Can you work these out from the model? Positions are in its coordinate system, mm. Round coordinates to 2 decimals unless told otherwise and drop trailing zeros. Write each loop counter-clockwise with the first axis right and the second up, starting at its lowest first coordinate (ties: lowest second). Pieces come first, ordered by that corner, then holes. Notation, with made-up numbers: (3, 21) - (42, 21) arc R18 ccw to (42, 49) - close; hole circle Ø5 at (69, 38). An arc over 180 degrees is marked (long way). One line per item, written item: value. Start each with the question number.
(1) I want a section at B-B on x = -35.5. List the corners of the cut face in (y, z) for me, plus the area to 3 significant figures.
(2) If I drill on L1, parallel to X at y = 2.4, z = -50; L2, parallel to Z at x = 51.5, y = 1.6; L3, parallel to Z at x = 17, y = 2.65, over which ranges is the centre line in solid material (lowest first)? Write a range as from..to.
(3) I want a section at A-A on y = 1.2. Give the number of separate pieces and of enclosed holes in the cut face, plus the area to 3 significant figures.
(4) I want a section at C-C on z = 21. List the corners of the cut face in (x, y) for me.
(5) I'm going to push flat-ended pins straight in: pin 1 Ø3 at (x, z) = (0, 0) entering from +Y; pin 2 Ø1 at (y, z) = (1, 41) entering from +X; pin 3 Ø1.5 at (y, z) = (1, -5.5) entering from -X; pin 4 Ø0.9 at (x, y) = (-87.5, 1) entering from -Z. Where does each tip first touch, or does it pass through?
from build123d import *

# Parameters (mm, degrees)
SKETCH_1_W            = 85
SKETCH_1_H            = 60
SKETCH_1_R            = 1.6
EXTRUDE_1_DEPTH       = 3
EXTRUDE_2_DEPTH       = 3
FILLET_1_R            = 20
FILLET_3_R            = 10
SKETCH_4_R            = 3.1
CUT_EXTRUDE_1_DEPTH   = 10
CUT_EXTRUDE_1_2_DEPTH = 10


with BuildPart() as part:
    # 草图1 → 凸台-拉伸1 (new body)
    with BuildSketch(Plane(origin=(0, 0, 0), x_dir=(1, 0, 0), z_dir=(0, 1, 0))):
        with Locations((32.5, 25)):
            Rectangle(SKETCH_1_W, SKETCH_1_H)
        with Locations(Location((0, 50, 0), (0, 0, 270))):
            Circle(SKETCH_1_R, mode=Mode.SUBTRACT)
        with Locations(Location((65, 50, 0), (0, 0, 90))):
            Circle(SKETCH_1_R, mode=Mode.SUBTRACT)
        with Locations(Location((65, 0, 0), (0, 0, 270))):
            Circle(SKETCH_1_R, mode=Mode.SUBTRACT)
        with Locations(Location((0, 0, 0), (0, 0, 90))):
            Circle(SKETCH_1_R, mode=Mode.SUBTRACT)
    extrude(amount=EXTRUDE_1_DEPTH)

    # 草图2 → 凸台-拉伸2 (add)
    with BuildSketch(Plane(origin=(0, 0, 0), x_dir=(1, 0, 0), z_dir=(0, 1, 0))):
        Polygon((-10, -5), (75, -5), (75, -25), (11.360389693, -88.639610307), (-58.172444533, -88.639610307), (-113.639610307, -88.639610307), (-157.279220614, -45), (-170.208152802, -32.071067812), (-130.208152802, -32.071067812), (-117.279220614, -45), (-10, -45), align=None)
    extrude(amount=EXTRUDE_2_DEPTH)

    # 圆角1
    fillet_1_edges = [part.edges().sort_by_distance(p)[0] for p in [
        (-10, 1.5, 45),
    ]]
    fillet(fillet_1_edges, radius=FILLET_1_R)

    # 圆角3
    fillet_3_edges = [part.edges().sort_by_distance(p)[0] for p in [
        (-130.208152802, 1.5, 32.071067812),
        (-170.208152802, 1.5, 32.071067812),
        (-113.639610307, 1.5, 88.639610307),
    ]]
    fillet(fillet_3_edges, radius=FILLET_3_R)

    # 草图4 → Cut-Extrude 1 (cut)
    with BuildSketch(Plane(origin=(0, 3, 0), x_dir=(1, 0, 0), z_dir=(0, 1, 0))):
        with Locations(Location((-146.066017178, -42.071067812, 0), (0, 0, 270))):
            Circle(SKETCH_4_R)
        with Locations(Location((-109.497474683, -78.639610307, 0), (0, 0, 270))):
            Circle(SKETCH_4_R)
    extrude(amount=-CUT_EXTRUDE_1_DEPTH, mode=Mode.SUBTRACT)

    # 草图5 → Cut-Extrude 1 2 (cut)
    with BuildSketch(Plane(origin=(0, 3, 0), x_dir=(1, 0, 0), z_dir=(0, 1, 0))):
        Polygon((25.202795796, 11.918524548), (12.121320344, 25), (25.202795796, 38.081475452), (23.081475452, 40.202795796), (7.878679656, 25), (23.081475452, 9.797204204), align=None)
        Polygon((40.202795796, 11.918524548), (27.121320344, 25), (40.202795796, 38.081475452), (38.081475452, 40.202795796), (22.878679656, 25), (38.081475452, 9.797204204), align=None)
        Polygon((55.202795796, 11.918524548), (42.121320344, 25), (55.202795796, 38.081475452), (53.081475452, 40.202795796), (37.878679656, 25), (53.081475452, 9.797204204), align=None)
    extrude(amount=-CUT_EXTRUDE_1_2_DEPTH, mode=Mode.SUBTRACT)


solid = part.part
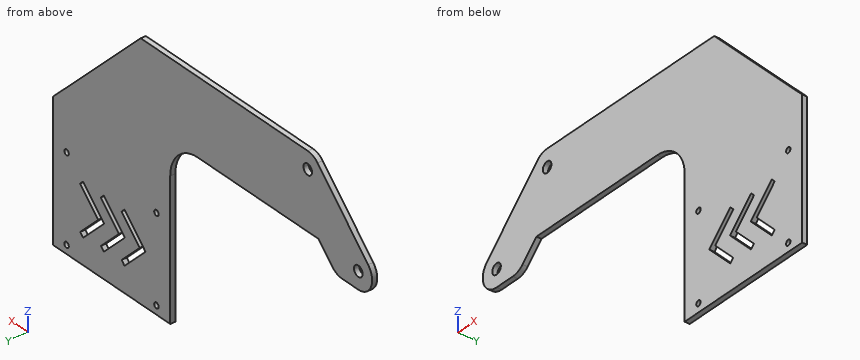
Established:
1. outline: (0, 45) - (3, 45) - (3, 88.64) - (0, 88.64) - close
1. area: 131 mm2
2. L1: -10..-1.6, 1.6..63.4, 66.6..75
2. L2: -55..-38.62, -34.38..-15.62, -11.38..48.5
2. L3: -55..-34.12, -29.88..-20.12, -15.88..83
3. separate pieces: 1
3. enclosed holes: 9
3. area: 15,700 mm2
4. outline: (-10, 0) - (75, 0) - (75, 3) - (-10, 3) - close
5. pin 1: through
5. pin 2: x = 59.5
5. pin 3: x = -10
5. pin 4: z = 45
